from build123d import *

# Parameters (mm, degrees)
SKETCH_1_W      = 155
SKETCH_1_H      = 125
EXTRUDE_1_DEPTH = 5
FILLET_1_R      = 10


with BuildPart() as part:
    # 草图1 → 凸台-拉伸1 (new body)
    with BuildSketch(Plane.XY):
        with Locations((77.5, 62.5)):
            Rectangle(SKETCH_1_W, SKETCH_1_H)
        with BuildLine():
            Line((11, 67.5), (144, 67.5))
            ThreePointArc((144, 67.5), (149, 62.5), (144, 57.5))
            Line((144, 57.5), (11, 57.5))
            ThreePointArc((11, 57.5), (6, 62.5), (11, 67.5))
        make_face(mode=Mode.SUBTRACT)
    extrude(amount=EXTRUDE_1_DEPTH)

    # 圆角1
    # the kernel refuses this fillet: 10 mm, written as the material it takes off along each edge
    with BuildSketch(Plane(origin=(0, 146.650635095, 5), x_dir=(0, 0, -1), z_dir=(0, -1, 0)), Plane(origin=(155, -21.650635095, 5), x_dir=(0, 0, -1), z_dir=(0, 1, 0))) as fillet_1_piece_1:
        with BuildLine():
            CenterArc((10, 8.660254038), FILLET_1_R, 180, 60)
            Line((0, 8.660254038), (-0.2, 8.660254038))
            Line((-0.2, 8.660254038), (-0.2, 0))
            Line((-0.2, 0), (0, -0.2))
            ThreePointArc((0, -0.2), (2.5, -0.2), (4.9, -0.173205081))
            Line((4.9, -0.173205081), (5, 0))
        make_face()
    extrude(amount=168.301270189, mode=Mode.SUBTRACT)
    with BuildSketch(Plane(origin=(-21.650635095, 0, 5), x_dir=(0, 0, -1), z_dir=(1, 0, 0)), Plane(origin=(176.650635095, 125, 5), x_dir=(0, 0, -1), z_dir=(-1, 0, 0))) as fillet_1_piece_2:
        with BuildLine():
            CenterArc((10, 8.660254038), FILLET_1_R, 180, 60)
            Line((0, 8.660254038), (-0.2, 8.660254038))
            Line((-0.2, 8.660254038), (-0.2, 0))
            Line((-0.2, 0), (0, -0.2))
            ThreePointArc((0, -0.2), (2.5, -0.2), (4.9, -0.173205081))
            Line((4.9, -0.173205081), (5, 0))
        make_face()
    extrude(amount=198.301270189, mode=Mode.SUBTRACT)


solid = part.part
For this review, take the finished solid that the model builds, in its own axes (mm). A direction names the side the tool comes from. Round coordinates to 2 decimals unless told otherwise and drop trailing zeros. Write each loop counter-clockwise with the first axis right and the second up, starting at its lowest first coordinate (ties: lowest second). Pieces come first, ordered by that corner, then holes. Notation, with made-up numbers: M 67.5,79.5 L 90.5,79.5 A38 ccw 90.5,117.5 Z; hole C 5,69 d1. An arc over 180 degrees is marked long. Write item = value, one per line. Start each with the question number.
(1) We need section C-C (y = 38). Give the boundary of the cut face in (x, z).
(2) We need section B-B (z = 3.15). Give the boundary of the cut face in (x, y).
(3) We need section A-A (x = 100). Give the boundary of the cut face in (y, z), then the cut area to 3 significant figures.
(4) The part is to be moulded in two halves that separate along X. For faces 1 (the face through (3.724, 63.375, 3.697)), 2 (the face through (6, 62.4, 2.5)), 3 (the face through (151.276, 61.625, 3.697)), say which applies: +X half, -X half, draft (parallel to the pull), parting line (faces both ways), or undercut.
(5) For faces 4 (the face through (149, 62.6, 2.5)), 5 (the face through (76, 77, 0)), list the 3-axis set-ups (+Z, -Z, +X, -X, +Y, -Y) from which the entire face can be reached by the end or side of a thin tool; tool diameter is ignored.
(6) Clearance check with flat-ended pins moving along their axes: pin 1 Ø2 at (x, z) = (22.5, 3.5) entering from +Y; pin 2 Ø2 at (x, z) = (52, 3) entering from -Y; pin 3 Ø1.5 at (y, z) = (86.5, 3) entering from -X. State where each tip first meets the part, or that it passes through.
(7) For line 1 along Y through (x, z) = (70, 2.7); line 2 along Y through (x, z) = (21.5, 3.65); line 3 along Z through (x, y) = (130, 117), list the stretches that pass through material, from the lowest coordinate up.
Results found:
q1.outline = M 0,0 L 155,0 A10 ccw 146.34,5 L 8.66,5 A10 ccw Z
q2.outline = M 2.87,2.87 L 152.13,2.87 L 152.13,122.13 L 2.87,122.13 Z; hole M 11,57.5 L 144,57.5 A5 ccw 144,67.5 L 11,67.5 A5 ccw Z
q3.outline = M 0,0 L 57.5,0 L 57.5,5 L 8.66,5 A10 ccw Z; M 67.5,0 L 125,0 A10 ccw 116.34,5 L 67.5,5 Z
q3.area = 550 mm²
q4.face_1 = -X half
q4.face_2 = undercut
q4.face_3 = +X half
q5.face_4 = +Z, -Z
q5.face_5 = -Z, +X, -X, +Y, -Y
q6.pin_1 = 122.95
q6.pin_2 = 1.52
q6.pin_3 = 1.77
q7.line_1 = 2.28 to 57.5, 67.5 to 122.72
q7.line_2 = 3.64 to 57.5, 67.5 to 121.36
q7.line_3 = 0 to 4.98
